from build123d import *

# Parameters (mm, degrees)
SKETCH1_W           = 139
SKETCH1_H           = 30
SKETCH1_R           = 1.6
SKETCH1_R_2         = 5.1
SKETCH1_R_3         = 3.75
SKETCH1_R_4         = 3.1
SKETCH1_R_5         = 1.25
SKETCH1_W_2         = 2.2
SKETCH1_H_2         = 1.1
SKETCH1_W_3         = 2.5
SKETCH1_H_3         = 1
SKETCH1_W_4         = 3.8
SKETCH1_H_4         = 1.9
BOSS_EXTRUDE1_DEPTH = 3


with BuildPart() as part:
    # Sketch1 → Boss-Extrude1 (new body)
    with BuildSketch(Plane.XY):
        with Locations((69.5, 15)):
            Rectangle(SKETCH1_W, SKETCH1_H)
        with Locations((4, 19.5)):
            Circle(SKETCH1_R, mode=Mode.SUBTRACT)
        with Locations((135, 19.5)):
            Circle(SKETCH1_R, mode=Mode.SUBTRACT)
        with Locations((124, 19.5)):
            Circle(SKETCH1_R, mode=Mode.SUBTRACT)
        with Locations((39.361239448, 15.906458033)):
            Circle(SKETCH1_R_2, mode=Mode.SUBTRACT)
        with Locations((63.522500572, 15.906458033)):
            Circle(SKETCH1_R_3, mode=Mode.SUBTRACT)
        with Locations((81.730883445, 15.906458033)):
            Circle(SKETCH1_R_4, mode=Mode.SUBTRACT)
        with Locations((108.399727047, 15.906458033)):
            Circle(SKETCH1_R_3, mode=Mode.SUBTRACT)
        with Locations((4, 5.895808563)):
            Circle(SKETCH1_R_5, mode=Mode.SUBTRACT)
        with Locations((124, 6.5)):
            Circle(SKETCH1_R, mode=Mode.SUBTRACT)
        with Locations((63.522500572, 9.656458033)):
            Rectangle(SKETCH1_W_2, SKETCH1_H_2, mode=Mode.SUBTRACT)
        with Locations((81.730883445, 9.906458033)):
            Rectangle(SKETCH1_W_3, SKETCH1_H_3, mode=Mode.SUBTRACT)
        with Locations((108.399727047, 8.406458033)):
            Rectangle(SKETCH1_W_4, SKETCH1_H_4, mode=Mode.SUBTRACT)
        with BuildLine():
            Line((16.505280772, 12.956458033), (20.632022828, 12.956458033))
            ThreePointArc((20.632022828, 12.956458033), (22.1686518, 15.906458033), (20.632022828, 18.856458033))
            Line((20.632022828, 18.856458033), (16.505280772, 18.856458033))
            ThreePointArc((16.505280772, 18.856458033), (14.9686518, 15.906458033), (16.505280772, 12.956458033))
        make_face(mode=Mode.SUBTRACT)
    extrude(amount=BOSS_EXTRUDE1_DEPTH)


solid = part.part
Check sheet for the modelled part. Datum: model origin and axes. Units: mm. A direction names the side the tool comes from. Round coordinates to 2 decimals unless told otherwise and drop trailing zeros. Loops run counter-clockwise (first coordinate to the right, second up) from the corner with the lowest first, then second, coordinate; pieces in that order, holes last.
1. Mould release check, pull along X, two halves, no side actions. Record for faces 1 (the flat face through (82, 9.406, 1)), 2 (the flat face through (139, 15, 1)), 3 (the flat face through (69, 0, 1)): released by +X, released by -X, zero draft, split by the parting line, or undercut.
2. Sectioned sample at B-B on x = 4. Record the boundary of the cut face in (y, z), and give its area (3 significant figures).
3. Sectioned sample at C-C on z = 2.3. Give the number of separate pieces and of enclosed holes in the cut face, and give its area (3 significant figures).
4. Set-up check for faces 4 (the flat face through (64, 10.206, 1)), 5 (the flat face through (69, 15, 3)): record each of +Z, -Z, +X, -X, +Y, -Y from which the full face is reachable in a straight line by a thin tool's end or side.
5. Gauge pin test, flat end, axial feed: pin 1 Ø12 at (x, y) = (123, 24) entering from -Z. Record the tip position at first contact, or that the pin passes through.
6. Scan lines: probe 1 along Y at (x, z) = (4, 1.8); probe 2 along Y at (x, z) = (124, 1); probe 3 along Y at (x, z) = (110.5, 0.3). Record each from-to range of solid material in increasing order.
7. Sectioned sample at A-A on x = 135. Record the boundary of the cut face in (y, z), and give its area (3 significant figures).
Recorded:
1. face 1: undercut
1. face 2: released by +X
1. face 3: zero draft
2. outline: (0, 0) - (4.65, 0) - (4.65, 3) - (0, 3) - close; (7.15, 0) - (17.9, 0) - (17.9, 3) - (7.15, 3) - close; (21.1, 0) - (30, 0) - (30, 3) - (21.1, 3) - close
2. area: 72.9 mm2
3. separate pieces: 1
3. enclosed holes: 13
3. area: 3,880 mm2
4. face 4: +Z, -Z
4. face 5: +Z, +X, -X, +Y, -Y
5. pin 1: stops at z = 0
6. probe 1: y = 0 to 4.65, 7.15 to 17.9, 21.1 to 30
6. probe 2: y = 0 to 4.9, 8.1 to 17.9, 21.1 to 30
6. probe 3: y = 0 to 12.8, 19.01 to 30
7. outline: (0, 0) - (17.9, 0) - (17.9, 3) - (0, 3) - close; (21.1, 0) - (30, 0) - (30, 3) - (21.1, 3) - close
7. area: 80.4 mm2
